Can you work these out from the model? Positions are in its coordinate system, mm. A direction names the side the tool comes from. Give positions to 0.01 mm unless a question says otherwise; leave off trailing zeros. Loops run counter-clockwise (first coordinate to the right, second up) from the corner with the lowest first, then second, coordinate; pieces in that order, holes last. Notation, with made-up numbers: M 43.25,-2 L 98.25,-2 A21 cw 98.25,12 Z; hole C -6.5,2.25 d10. An arc over 180 degrees is marked long. Answer as a JSON object with one key per item and string values.
```python
from build123d import *

# Parameters (mm, degrees)
F0_R     = 19.05
F1_DEPTH = 63.5
F2_R     = 5.5626
F3_DEPTH = 4.7752
F4_DEPTH = 4.7752
F5_DEPTH = 15.875
F6_DEPTH = 20.6502
F7_R     = 5.5626
F8_DEPTH = 20.6502
F9_DEPTH = 15.875


with BuildPart() as f1:
    # F0 (on Front) → F1 (new body)
    with BuildSketch(Plane.XZ):
        with BuildLine():
            Line((69.85, 28.575), (0, 28.575))
            ThreePointArc((0, 28.575), (-22.5905210348, -17.49854235), (27.6676247795, -7.14375))
            Line((27.6676247795, -7.14375), (27.6676247795, 3.175))
            ThreePointArc((27.6676247795, 3.175), (30.4574326887, 9.9101920908), (37.1926247795, 12.7))
            Line((37.1926247795, 12.7), (69.85, 12.7))
            Line((69.85, 12.7), (69.85, 28.575))
        make_face()
        Circle(F0_R, mode=Mode.SUBTRACT)
    extrude(amount=F1_DEPTH)

    # F2 (on face) → F3 (join)
    with BuildSketch(Plane.XY.offset(28.575)):
        with BuildLine():
            Line((90.4493554441, -20.7222785358), (57.0991554441, -1.6722785358))
            ThreePointArc((57.0991554441, -1.6722785358), (44.4246284085, -1.7161647377), (38.1, -12.7))
            Line((38.1, -12.7), (38.1, -50.8))
            ThreePointArc((38.1, -50.8), (44.4246284085, -61.7838352623), (57.0991554441, -61.8277214642))
            Line((57.0991554441, -61.8277214642), (90.4493554441, -42.7777214642))
            ThreePointArc((90.4493554441, -42.7777214642), (96.8502, -31.75), (90.4493554441, -20.7222785358))
        make_face()
        with Locations((50.8, -50.8)):
            Circle(F2_R, mode=Mode.SUBTRACT)
        with Locations((50.8, -12.7)):
            Circle(F2_R, mode=Mode.SUBTRACT)
        with Locations((84.1502, -31.75)):
            Circle(F2_R, mode=Mode.SUBTRACT)
        with Locations((84.1502, -31.75)):
            Circle(F2_R)
    extrude(amount=F3_DEPTH)

    # F2 (on face) → F4 (join)
    with BuildSketch(Plane.XY.offset(28.575)):
        with BuildLine():
            Line((90.4493554441, -20.7222785358), (57.0991554441, -1.6722785358))
            ThreePointArc((57.0991554441, -1.6722785358), (44.4246284085, -1.7161647377), (38.1, -12.7))
            Line((38.1, -12.7), (38.1, -50.8))
            ThreePointArc((38.1, -50.8), (44.4246284085, -61.7838352623), (57.0991554441, -61.8277214642))
            Line((57.0991554441, -61.8277214642), (90.4493554441, -42.7777214642))
            ThreePointArc((90.4493554441, -42.7777214642), (96.8502, -31.75), (90.4493554441, -20.7222785358))
        make_face()
        with Locations((50.8, -50.8)):
            Circle(F2_R, mode=Mode.SUBTRACT)
        with Locations((50.8, -12.7)):
            Circle(F2_R, mode=Mode.SUBTRACT)
        with Locations((84.1502, -31.75)):
            Circle(F2_R, mode=Mode.SUBTRACT)
    extrude(amount=F4_DEPTH)

    # F5 (cut, through all): faces of the model
    f5_faces = [f1.faces().sort_by_distance(p)[0] for p in [
        (64.480850076, -2.9493294549, 28.575),
        (64.480850076, -60.5506705451, 28.575),
    ]]
    extrude(f5_faces, amount=-F5_DEPTH, mode=Mode.SUBTRACT)

    # F6 (cut): faces of the model
    f6_faces = [f1.faces().sort_by_distance(p)[0] for p in [
        (50.8, -12.7, 28.575),
        (50.8, -50.8, 28.575),
    ]]
    extrude(f6_faces, amount=-F6_DEPTH, mode=Mode.SUBTRACT)

    # F7 (on face) → F8 (cut)
    with BuildSketch(Plane.XY.offset(33.3502)):
        with Locations((84.1502, -31.75)):
            Circle(F7_R)
    extrude(amount=-F8_DEPTH, mode=Mode.SUBTRACT)

    # F9 (add, through all): a face of the model
    f9_faces = [f1.faces().sort_by_distance(p)[0] for p in [
        (96.3203574662, -31.75, 28.575),
    ]]
    extrude(f9_faces, amount=F9_DEPTH)


solid = f1.part
```
1) Please list where these lines run through material, in increasing order: line 1 along Z through (x, y) = (0, -11.5) (3 decimals); line 2 along X through (y, z) = (-38.5, 16); line 3 along Z through (x, y) = (66, -9.5). Write a range as from..to.
Answer list:
{"line 1": "-28.575..-19.05, 19.05..28.575", "line 2": "-23.68..-10.34, 10.34..94.91", "line 3": "12.7..33.35"}
2) Will these pins go through, and if not, where does the flat tip stop? pin 1 Ø18 at (x, y) = (77, -46) entering from -Z; pin 2 Ø10 at (x, y) = (84.15, -31.75) entering from +Z; pin 3 Ø3 at (y, z) = (-22.5, 9.5) entering from +X; pin 4 Ø8.5 at (y, z) = (-16.5, -2.5) entering from +X.
Answer list:
{"pin 1": "z = 12.7", "pin 2": "through", "pin 3": "x = 31.76", "pin 4": "x = 27.67"}
3) For faces 1 (the cylindrical face through (50.205, -0.014, 29.764)), 2 (the flat face through (38.1, -31, 31)), 3 (the cylindrical face through (49.834, -63.463, 29.764)), 4 (the flat face through (73.541, -52.436, 23.17)), 5 (the flat face through (60, -31, 12.7)), which set-ups out of +Z, -Z, +X, -X, +Y, -Y let a thin tool reach every point of the face, with its end or its side?
Answer list:
{"face 1": "+Z, +Y", "face 2": "+Z, -X, +Y, -Y", "face 3": "+Z, -Y", "face 4": "+Z, -Z, +X, -Y", "face 5": "-Z, +X, +Y, -Y"}
4) If we mould it in two halves opening along X, with no side actions, what happens to faces 6 (the flat face through (19, -63.5, 7)), 7 (the flat face through (74.01, -11.33, 23.17)), 8 (the cylindrical face through (-15.12, -31.31, -11.59))? For each: +X half, -X half, draft (parallel to the pull), parting line (faces both ways), or undercut.
Answer list:
{"face 6": "draft", "face 7": "+X half", "face 8": "undercut"}
5) Suppose I cut it at A-A, the plane y = -31.75. Write out the boundary of the cut face in (x, z) (3 decimals).
Answer list:
{"outline": "M 0,28.575 A28.575 ccw long 27.668,-7.144 L 27.668,3.175 A9.525 cw 37.193,12.7 L 78.588,12.7 L 78.588,33.35 L 38.1,33.35 L 38.1,28.575 Z; M 89.713,12.7 L 96.85,12.7 L 96.85,33.35 L 89.713,33.35 Z; hole C 0,0 d38.1"}
6) Suppose I cut it at C-C, the plane x = -5. Write out the boundary of the cut face in (y, z).
Answer list:
{"outline": "M -63.5,-28.13 L 0,-28.13 L 0,-18.38 L -63.5,-18.38 Z; M -63.5,18.38 L 0,18.38 L 0,28.13 L -63.5,28.13 Z"}
7) Suppose I cut it at D-D, the plane y = -11. Write out the boundary of the cut face in (x, z) (3 decimals).
Answer list:
{"outline": "M 0,28.575 A28.575 ccw long 27.668,-7.144 L 27.668,3.175 A9.525 cw 37.193,12.7 L 45.504,12.7 L 45.504,33.35 L 38.214,33.35 L 38.214,28.575 Z; M 56.096,12.7 L 73.429,12.7 L 73.429,33.35 L 56.096,33.35 Z; hole C 0,0 d38.1"}
8) Suppose I cut it at B-B, the plane z = 0. Write out the boundary of the cut face in (x, y) (3 decimals).
Answer list:
{"outline": "M -28.575,-63.5 L -19.05,-63.5 L -19.05,0 L -28.575,0 Z; M 19.05,-63.5 L 27.668,-63.5 L 27.668,0 L 19.05,0 Z"}
